Could you check a few things on this model? Use its own coordinates, in mm. A direction names the side the tool comes from. Coordinates: 2 decimals unless noted, no trailing zeros. Loops run counter-clockwise (first coordinate to the right, second up) from the corner with the lowest first, then second, coordinate; pieces in that order, holes last. Notation, with made-up numbers: (-29, 45) -> (-5, 45) arc R19 cw to (-5, 62) -> close; hole circle Ø7 at (70.25, -39.75). An arc over 180 degrees is marked (long way). One line per question, with ' | ' between items.
from build123d import *

# Parameters (mm, degrees)
F0_W     = 15.8
F0_H     = 63.72
F0_R     = 2.43
F1_DEPTH = 9.71
F2_DEPTH = 1.86


with BuildPart() as f1:
    # F0 (on Top) → F1 (new body)
    with BuildSketch(Plane.XY):
        with Locations((-51.7484200151, -3.5033859313)):
            Rectangle(F0_W, F0_H)
        with Locations((-55.9428147972, -28.2833859313)):
            Circle(F0_R, mode=Mode.SUBTRACT)
        with Locations((-55.9428147972, -21.2033859313)):
            Circle(F0_R, mode=Mode.SUBTRACT)
        with Locations((-55.9428147972, -14.1233859313)):
            Circle(F0_R, mode=Mode.SUBTRACT)
        with Locations((-55.9428147972, -7.0433859313)):
            Circle(F0_R, mode=Mode.SUBTRACT)
        with Locations((-47.8049702942, -28.2833859313)):
            Circle(F0_R, mode=Mode.SUBTRACT)
        with Locations((-47.8049702942, -21.2033859313)):
            Circle(F0_R, mode=Mode.SUBTRACT)
        with Locations((-47.8049702942, -14.1233859313)):
            Circle(F0_R, mode=Mode.SUBTRACT)
        with Locations((-47.8049702942, -7.0433859313)):
            Circle(F0_R, mode=Mode.SUBTRACT)
        with Locations((-55.9428147972, 0)):
            Circle(F0_R, mode=Mode.SUBTRACT)
        with Locations((-55.9428147972, 7.1166140687)):
            Circle(F0_R, mode=Mode.SUBTRACT)
        with Locations((-55.9428147972, 14.1966140687)):
            Circle(F0_R, mode=Mode.SUBTRACT)
        with Locations((-55.9428147972, 21.2766140687)):
            Circle(F0_R, mode=Mode.SUBTRACT)
        with Locations((-47.8049702942, 0)):
            Circle(F0_R, mode=Mode.SUBTRACT)
        with Locations((-47.8049702942, 7.1166140687)):
            Circle(F0_R, mode=Mode.SUBTRACT)
        with Locations((-47.8049702942, 14.1966140687)):
            Circle(F0_R, mode=Mode.SUBTRACT)
        with Locations((-47.8049702942, 21.2766140687)):
            Circle(F0_R, mode=Mode.SUBTRACT)
        with Locations((-55.9428147972, 21.2766140687)):
            Circle(F0_R)
        with Locations((-55.9428147972, 14.1966140687)):
            Circle(F0_R)
        with Locations((-55.9428147972, 7.1166140687)):
            Circle(F0_R)
        with Locations((-55.9428147972, 0)):
            Circle(F0_R)
        with Locations((-55.9428147972, -7.0433859313)):
            Circle(F0_R)
        with Locations((-55.9428147972, -14.1233859313)):
            Circle(F0_R)
        with Locations((-55.9428147972, -21.2033859313)):
            Circle(F0_R)
        with Locations((-55.9428147972, -28.2833859313)):
            Circle(F0_R)
        with Locations((-47.8049702942, -28.2833859313)):
            Circle(F0_R)
        with Locations((-47.8049702942, -21.2033859313)):
            Circle(F0_R)
        with Locations((-47.8049702942, -14.1233859313)):
            Circle(F0_R)
        with Locations((-47.8049702942, -7.0433859313)):
            Circle(F0_R)
        with Locations((-47.8049702942, 0)):
            Circle(F0_R)
        with Locations((-47.8049702942, 7.1166140687)):
            Circle(F0_R)
        with Locations((-47.8049702942, 14.1966140687)):
            Circle(F0_R)
        with Locations((-47.8049702942, 21.2766140687)):
            Circle(F0_R)
    extrude(amount=-F1_DEPTH)

    # F0 (on Top) → F2 (join)
    with BuildSketch(Plane.XY):
        with Locations((-55.9428147972, 21.2766140687)):
            Circle(F0_R)
        with Locations((-55.9428147972, 14.1966140687)):
            Circle(F0_R)
        with Locations((-55.9428147972, 7.1166140687)):
            Circle(F0_R)
        with Locations((-55.9428147972, 0)):
            Circle(F0_R)
        with Locations((-55.9428147972, -7.0433859313)):
            Circle(F0_R)
        with Locations((-55.9428147972, -14.1233859313)):
            Circle(F0_R)
        with Locations((-55.9428147972, -21.2033859313)):
            Circle(F0_R)
        with Locations((-55.9428147972, -28.2833859313)):
            Circle(F0_R)
        with Locations((-47.8049702942, -28.2833859313)):
            Circle(F0_R)
        with Locations((-47.8049702942, -21.2033859313)):
            Circle(F0_R)
        with Locations((-47.8049702942, -14.1233859313)):
            Circle(F0_R)
        with Locations((-47.8049702942, -7.0433859313)):
            Circle(F0_R)
        with Locations((-47.8049702942, 0)):
            Circle(F0_R)
        with Locations((-47.8049702942, 7.1166140687)):
            Circle(F0_R)
        with Locations((-47.8049702942, 14.1966140687)):
            Circle(F0_R)
        with Locations((-47.8049702942, 21.2766140687)):
            Circle(F0_R)
    extrude(amount=F2_DEPTH)


solid = f1.part
1) On a 3-axis mill with a long thin cutter (end or side, diameter ignored), from which of +Z, -Z, +X, -X, +Y, -Y can I reach the whole of each face in a straight line? I mean faces 1 (the face through (-56, -28, 1.86)), 2 (the face through (-53.625, -27.553, 0.917)). Say none if no direction works.
Data:
face 1: +Z, +X, -X, +Y, -Y | face 2: +Z
2) If we section it at A-A on y = 0: Please give me the cut outline in (x, z), and give its area (3 significant figures).
Data:
outline: (-59.65, -9.71) -> (-43.85, -9.71) -> (-43.85, 0) -> (-45.37, 0) -> (-45.37, 1.86) -> (-50.23, 1.86) -> (-50.23, 0) -> (-53.51, 0) -> (-53.51, 1.86) -> (-58.37, 1.86) -> (-58.37, 0) -> (-59.65, 0) -> close | area: 171 mm²
3) I'm going to push a flat-ended pin straight in: pin 1 Ø1 at (x, y) = (-50, 3) entering from +Z. Where does the tip first touch, or does it pass through?
Data:
pin 1: z = 0
4) I need wall thicknesses on line 1 along Z through (x, y) = (-44.75, 2.5); line 2 along X through (y, z) = (-23, 0.25). Which ranges of each line are inside material? Lowest first, please. Write a range as from..to.
Data:
line 1: -9.71..0 | line 2: -57.58..-54.31, -49.44..-46.17
5) If we section it at B-B on z = 0.75: Give the number of separate pieces and of enclosed holes in the cut face, and give its area (3 significant figures).
Data:
separate pieces: 16 | enclosed holes: 0 | area: 297 mm²
6) If we section it at C-C on y = 9: Please give me the cut outline in (x, z).
Data:
outline: (-59.65, -9.71) -> (-43.85, -9.71) -> (-43.85, 0) -> (-46.27, 0) -> (-46.27, 1.86) -> (-49.34, 1.86) -> (-49.34, 0) -> (-54.41, 0) -> (-54.41, 1.86) -> (-57.48, 1.86) -> (-57.48, 0) -> (-59.65, 0) -> close
7) We'd pull the mould along Y, two halves only. Please class faces 3 (the face through (-52, -3, 0)), 4 (the face through (-48, 0, 1.86)), 5 (the face through (-52, -35.363, -5)): pulls with the +Y half, pulls with the -Y half, needs draft (parallel to the pull), parting line crosses it, or undercut.
Data:
face 3: undercut | face 4: needs draft | face 5: pulls with the -Y half
